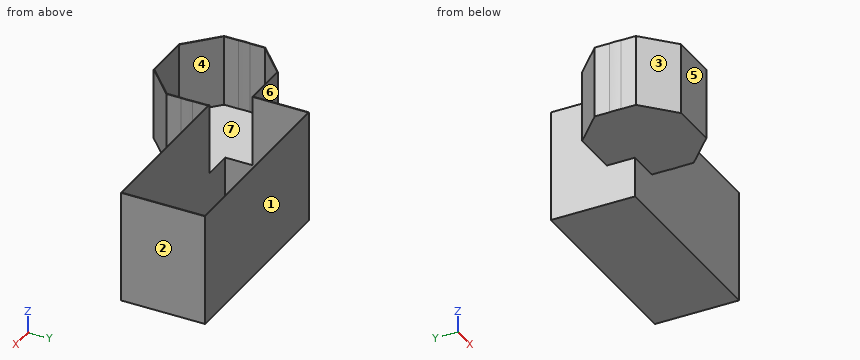
```python
from build123d import *

# Parameters (mm, degrees)
F1_W     = 88.9
F1_H     = 38.1
F2_DEPTH = 50.8
F3_DEPTH = 32.512
F4_T     = -0.254


with BuildPart() as f2:
    # F1 (on Top) → F2 (new body)
    with BuildSketch(Plane.XY):
        with Locations((-49.5874881029, 28.6405186608)):
            Rectangle(F1_W, F1_H)
    extrude(amount=-F2_DEPTH)

    # F0 (on Top) → F3 (join)
    with BuildSketch(Plane.XY):
        with BuildLine():
            Line((-129.0890981385, -2.6270174623), (-129.0890981385, 2.6270174623))
            ThreePointArc((-129.0890981385, 2.6270174623), (-129.2282210844, 0), (-129.0890981385, -2.6270174623))
        make_face()
        Polygon((-129.0890981385, 9.3266623309), (-129.0890981385, 2.6270174623), (-129.0890981385, -2.6270174623), (-129.0890981385, -9.3266623309), (-115.0795637781, -22.4417199168), (-93.6325612334, -22.4417199168), (-79.623026873, -9.3266623309), (-79.623026873, -2.6270174623), (-79.623026873, 2.6270174623), (-79.623026873, 9.3266623309), (-93.6325612334, 22.4417199168), (-115.0795637781, 22.4417199168), align=None)
        with BuildLine():
            ThreePointArc((-79.623026873, -2.6270174623), (-79.4839039271, 0), (-79.623026873, 2.6270174623))
            Line((-79.623026873, 2.6270174623), (-79.623026873, -2.6270174623))
        make_face()
    extrude(amount=-F3_DEPTH)

    # F4
    f4_openings = [f2.faces().sort_by_distance(p)[0] for p in [
        (-68.590003, 18.592115, 0),
    ]]
    offset(amount=F4_T, openings=f4_openings, kind=Kind.INTERSECTION)


solid = f2.part
```
Build history of the part. All positions in model axes, mm. Face numbers are marked on the shaded views. A direction names the side the tool comes from. Give positions to 0.01 mm unless a question says otherwise; leave off trailing zeros. Order: outer loops, then holes, each group sorted by start corner. A loop starts at its lowest first (then second) coordinate and runs counter-clockwise, first axis right, second up. Notation, with made-up numbers: M -31.5,40 L -19.5,40 A21 ccw -19.5,60 Z; hole C 11.5,46 d11. An arc over 180 degrees is marked long. Write item = value, one per line. Start each with the question number.
(1) Slice it at B-B on y = 0. Write the cut outline in (x, z), plus the area to 3 significant figures.
(2) Slice it at C-C on x = -103.5. Write the cut outline in (y, z), plus the area to 3 significant figures.
(3) Which spindle directions (+Z, -Z, +X, -X, +Y, -Y) get a long thin tool onto all of the face, cutting with end or side? Do the marked faces 5, 6 and 7. Say none if no direction does.
(4) Pin check, flat tips, straight feed: pin 1 Ø19 at (x, y) = (-48, 30) entering from +Z; pin 2 Ø5.5 at (y, z) = (4.5, -23.5) entering from +X; pin 3 Ø5 at (y, z) = (13, -14.5) entering from -X. Stop position of each tip, or through.
(5) Probe L1, parallel to Y at x = -104.5, z = -7; L2, parallel to Y at x = -83, z = -33.5; L3, parallel to X at y = 15, z = -39. List the from-to ranges inside material, lowest first. Write a range as [from, to].
(6) Two-plate mould, pull along Y, no slides. Class the marked faces 1, 2, 3 and 4: released by +Y, released by -Y, zero draft, split by the parting line, or undercut.
(7) Slice it at D-D on y = 17. Write the cut outline in (x, z).
Responses:
q1.outline = M -129.23,-32.51 L -79.48,-32.51 L -79.48,0 L -79.74,0 L -79.74,-32.26 L -128.97,-32.26 L -128.97,0 L -129.23,0 Z
q1.area = 29.0 mm2
q2.outline = M -22.44,-32.51 L 22.44,-32.51 L 22.44,0 L 22.19,0 L 22.19,-32.26 L -22.19,-32.26 L -22.19,0 L -22.44,0 Z
q2.area = 27.8 mm2
q3.face_5 = +Z, -Z, +X, -X, -Y
q3.face_6 = +Z, -Z, -X, +Y
q3.face_7 = +Z
q4.pin_1 = -50.55
q4.pin_2 = -79.55
q4.pin_3 = -127.84
q5.L1 = [-22.44, -22.19], [22.19, 22.44]
q5.L2 = [9.59, 9.84], [47.44, 47.69]
q5.L3 = [-94.04, -93.78], [-5.39, -5.14]
q6.face_1 = released by +Y
q6.face_2 = zero draft
q6.face_3 = released by -Y
q6.face_4 = undercut
q7.outline = M -120.89,-32.51 L -94.04,-32.51 L -94.04,-50.8 L -5.14,-50.8 L -5.14,0 L -5.39,0 L -5.39,-50.55 L -93.78,-50.55 L -93.78,-32.26 L -120.52,-32.26 L -120.52,0 L -120.89,0 Z
